Build history of the part. All positions in model axes, mm. A direction names the side the tool comes from. Give positions to 0.01 mm unless a question says otherwise; leave off trailing zeros. Order: outer loops, then holes, each group sorted by start corner. A loop starts at its lowest first (then second) coordinate and runs counter-clockwise, first axis right, second up. Notation, with made-up numbers: (29, 17.25) - (73, 17.25) arc R7 ccw to (73, 29.25) - close; hole circle Ø11 at (1.25, 74). An arc over 180 degrees is marked (long way). Write each question's results on one line, items separated by ' | '. Start each with the question number.
from build123d import *

# Parameters (mm, degrees)
SKETCH1_R                = 140
SKETCH1_R_2              = 97
BOSS_EXTRUDE1_DEPTH      = 112.5
SKETCH2_R                = 23.5
BOSS_EXTRUDE2_DEPTH      = 32
CIRPATTERN1_COUNT        = 3
MIRROR1_COPY_1_SKETCH_R  = 23.5
MIRROR1_COPY_1_DEPTH     = 32
MIRROR1_COPY_2_SKETCH_R  = 23.5
MIRROR1_COPY_2_DEPTH     = 32
BOSS_EXTRUDE3_REACH      = 489.344
BOSS_EXTRUDE3_END_RADIUS = 140
BOSS_EXTRUDE3_START      = -165
SKETCH3_R                = 100
BOSS_EXTRUDE4_REACH      = 499.344
BOSS_EXTRUDE4_END_RADIUS = 140
BOSS_EXTRUDE4_START      = 175
SKETCH4_R                = 37.5
SKETCH5_R                = 50
CUT_EXTRUDE1_DEPTH       = 25
SKETCH6_R                = 28.1
CUT_EXTRUDE2_DEPTH       = 310
SKETCH9_R                = 10.15
CUT_EXTRUDE3_DEPTH       = 15
CIRPATTERN2_COUNT        = 3


with BuildPart() as part:
    # Sketch1 → Boss-Extrude1 (new, symmetric)
    with BuildSketch(Plane(origin=(0, 0, 0), x_dir=(1, 0, 0), z_dir=(0, 1, 0))):
        with Locations(Location((0, 0, 0), (0, 0, 270))):
            Circle(SKETCH1_R)
        with Locations(Location((0, 0, 0), (0, 0, 270))):
            Circle(SKETCH1_R_2, mode=Mode.SUBTRACT)
    extrude(amount=BOSS_EXTRUDE1_DEPTH, both=True)

    # Sketch2 → Boss-Extrude2 (add)
    with BuildSketch(Plane(origin=(0, 112.5, 0), x_dir=(1, 0, 0), z_dir=(0, 1, 0))):
        with BuildLine():
            Line((175, 50), (130.766968306, 50))
            ThreePointArc((130.766968306, 50), (140, 0), (130.766968306, -50))
            Line((130.766968306, -50), (175, -50))
            ThreePointArc((175, -50), (225, 0), (175, 50))
        make_face()
        with Locations(Location((175, 0, 0), (0, 0, 270))):
            Circle(SKETCH2_R, mode=Mode.SUBTRACT)
    boss_extrude2 = extrude(amount=-BOSS_EXTRUDE2_DEPTH)

    # CirPattern1: Boss-Extrude2 ×3 about axis
    cirpattern1_axis = Axis((0, 0, 0), (0, 1, 0))
    for i in range(1, CIRPATTERN1_COUNT):
        add(boss_extrude2.rotate(cirpattern1_axis, i * 360 / CIRPATTERN1_COUNT))

    # Mirror1: Boss-Extrude2 across plane
    add(boss_extrude2.mirror(Plane.ZX))

    # Mirror1 copy 1 sketch → Mirror1 copy 1 (add)
    with BuildSketch(Plane(origin=(0, -112.5, 0), x_dir=(-0.4999999999999998, 0, -0.8660254037844387), z_dir=(0, -1, 0))):
        with BuildLine():
            Line((175, -50), (130.766968306, -50))
            ThreePointArc((130.766968306, -50), (140, 0), (130.766968306, 50))
            Line((130.766968306, 50), (175, 50))
            ThreePointArc((175, 50), (225, 0), (175, -50))
        make_face()
        with Locations((175, 0)):
            Circle(MIRROR1_COPY_1_SKETCH_R, mode=Mode.SUBTRACT)
    extrude(amount=-MIRROR1_COPY_1_DEPTH)

    # Mirror1 copy 2 sketch → Mirror1 copy 2 (add)
    with BuildSketch(Plane(origin=(0, -112.5, 0), x_dir=(-0.5000000000000004, 0, 0.8660254037844384), z_dir=(0, -1, 0))):
        with BuildLine():
            Line((175, -50), (130.766968306, -50))
            ThreePointArc((130.766968306, -50), (140, 0), (130.766968306, 50))
            Line((130.766968306, 50), (175, 50))
            ThreePointArc((175, 50), (225, 0), (175, -50))
        make_face()
        with Locations((175, 0)):
            Circle(MIRROR1_COPY_2_SKETCH_R, mode=Mode.SUBTRACT)
    extrude(amount=-MIRROR1_COPY_2_DEPTH)

    # Boss-Extrude3: up to this cylinder (the profile starts outside it)
    boss_extrude3_end = Plane(origin=(0, 0, 0), z_dir=(0, -1, 0)) * Cylinder(BOSS_EXTRUDE3_END_RADIUS, 1259.688, mode=Mode.PRIVATE)
    # Sketch3 → Boss-Extrude3 (add, up to the surface)
    with BuildSketch(Plane(origin=(0, 0, 0), x_dir=(0, 0, -1), z_dir=(1, 0, 0)).offset(BOSS_EXTRUDE3_START), mode=Mode.PRIVATE) as boss_extrude3_sk1:
        with Locations(Location((0, 0, 0), (0, 0, 180))):
            Circle(SKETCH3_R)
    boss_extrude3_tool1 = extrude(boss_extrude3_sk1.sketch, amount=BOSS_EXTRUDE3_REACH, mode=Mode.PRIVATE) - boss_extrude3_end
    add(boss_extrude3_tool1.solids().sort_by_distance((-165, 0, 0))[0])

    # Boss-Extrude4: up to this cylinder (the profile starts outside it)
    boss_extrude4_end = Plane(origin=(0, 0, 0), z_dir=(0, -1, 0)) * Cylinder(BOSS_EXTRUDE4_END_RADIUS, 1279.688, mode=Mode.PRIVATE)
    # Sketch4 → Boss-Extrude4 (add, up to the surface)
    with BuildSketch(Plane(origin=(0, 0, 0), x_dir=(0, 0, -1), z_dir=(1, 0, 0)).offset(BOSS_EXTRUDE4_START), mode=Mode.PRIVATE) as boss_extrude4_sk1:
        Circle(SKETCH4_R)
    boss_extrude4_tool1 = extrude(boss_extrude4_sk1.sketch, amount=-BOSS_EXTRUDE4_REACH, mode=Mode.PRIVATE) - boss_extrude4_end
    add(boss_extrude4_tool1.solids().sort_by_distance((175, 0, 0))[0])

    # Sketch5 → Cut-Extrude1 (cut)
    with BuildSketch(Plane.ZY.offset(165)):
        Circle(SKETCH5_R)
    extrude(amount=-CUT_EXTRUDE1_DEPTH, mode=Mode.SUBTRACT)

    # Sketch6 → Cut-Extrude2 (cut)
    with BuildSketch(Plane.ZY.offset(165)):
        Circle(SKETCH6_R)
    extrude(amount=-CUT_EXTRUDE2_DEPTH, mode=Mode.SUBTRACT)

    # Sketch9 → Cut-Extrude3 (cut)
    with BuildSketch(Plane.ZY.offset(165)):
        with Locations((0, 75)):
            Circle(SKETCH9_R)
    cut_extrude3 = extrude(amount=-CUT_EXTRUDE3_DEPTH, mode=Mode.SUBTRACT)

    # CirPattern2: Cut-Extrude3 ×3 about axis
    cirpattern2_axis = Axis((0, 0, 0), (1, 0, 0))
    for i in range(1, CIRPATTERN2_COUNT):
        add(cut_extrude3.rotate(cirpattern2_axis, i * 360 / CIRPATTERN2_COUNT), mode=Mode.SUBTRACT)


solid = part.part
Item 1: Which spindle directions (+Z, -Z, +X, -X, +Y, -Y) get a long thin tool onto all of the face, cutting with end or side? Do faces 1 (the flat face through (-150, -38, -65)), 2 (the flat face through (-119.9, -96.72, -107.67)), 3 (the cylindrical face through (118.05, 1.58, 75.26)), 4 (the flat face through (153, 97, 50)). Say none if no direction does.
Item 2: Flat gauge pins, fed straight in: pin 1 Ø1.5 at (x, y) = (121, 34) entering from -Z; pin 2 Ø12 at (x, y) = (55.5, -81.5) entering from +Z; pin 3 Ø3 at (y, z) = (-71, -117.5) entering from -X. Where does each tip first touch, or does it go through?
Item 3: Probe line 1 along Y through (x, z) = (150, -21); line 2 along Z through (x, y) = (-114, 93.5) (3 decimals); line 3 along Y through (x, z) = (-59.5, 138.5). List the from-to ranges inside material, lowest first. Write a range as from..to.
Item 4: Cut at B-B, the plane x = -87.5. Count the separate pieces of the cut face and the enclosed holes in it, then the cut area to 3 significant figures.
Item 5: Cut at C-C, the plane y = 0. List the corners of the cut face in (x, z), then the cut area to 3 significant figures.
Item 6: Two-plate mould, pull along Z, no slides. Class faces 5 (the flat face through (153, -97, -50)), 6 (the flat face through (-99, -80.5, -173)), 7 (the cylindrical face through (224.988, 96.724, 1.099)), 8 (the cylindrical face through (198.3, 96.72, -3.06)): +Z half, -Z half, draft (parallel to the pull), parting line (faces both ways), or undercut.
Item 7: Cut at A-A, the plane x = 10. List the corners of the cut face in (y, z).
Values found:
1) face 1: -X | face 2: -X, -Y | face 3: none | face 4: +Z, +X, +Y, -Y
2) pin 1: stops at z = -71.69 | pin 2: stops at z = 130.96 | pin 3: stops at x = -78.38
3) line 1: y = -112.5..-80.5, -31.07..31.07, 80.5..112.5 | line 2: z = -193.954..-97.454, -81.265..81.265, 97.454..193.954 | line 3: y = -112.5..-80.5, 80.5..112.5
4) separate pieces: 6 | enclosed holes: 0 | area: 36,100 mm2
5) outline: (-165, -100) - (-97.98, -100) arc R140 ccw to (134.88, -37.5) - (175, -37.5) - (175, 37.5) - (134.88, 37.5) arc R140 ccw to (-97.98, 100) - (-165, 100) - (-165, 50) - (-140, 50) - (-140, 28.1) - (-92.84, 28.1) arc R97 cw to (92.84, 28.1) - (145, 28.1) - (145, -28.1) - (92.84, -28.1) arc R97 cw to (-92.84, -28.1) - (-140, -28.1) - (-140, -50) - (-165, -50) - close | area: 34,600 mm2
6) face 5: -Z half | face 6: draft | face 7: parting line | face 8: undercut
7) outline: (-112.5, -139.64) - (112.5, -139.64) - (112.5, -96.48) - (-112.5, -96.48) - close; (-112.5, 96.48) - (112.5, 96.48) - (112.5, 139.64) - (-112.5, 139.64) - close
